CAD build for the part. Positions are in the model's coordinates, mm. A direction names the side the tool comes from. Coordinates: 2 decimals unless noted, no trailing zeros. Loops run counter-clockwise (first coordinate to the right, second up) from the corner with the lowest first, then second, coordinate; pieces in that order, holes last. Notation, with made-up numbers: (-16, 35.5) - (20, 35.5) arc R27 ccw to (20, 73.5) - close; hole circle Ø9 at (-13.5, -34.5). An arc over 180 degrees is marked (long way). Put each result on its own line as item: value.
Autodesk Inventor part; units mm, degrees
ref_plane "YZ Plane" through (0, 0, 0) normal (1, 0, 0) x (0, 1, 0)
ref_plane "XZ Plane" through (0, 0, 0) normal (0, 1, 0) x (-1, 0, 0)
ref_plane "XY Plane" through (0, 0, 0) normal (0, 0, 1) x (1, 0, 0)
sketch "スケッチ1" plane through (0, 0, 0) normal (0, 0, 1) x (1, 0, 0)
  line L0 (29.75, 17.5) -> (29.75, -17.5)
  line L1 (29.75, -17.5) -> (-29.75, -17.5)
  line L2 (-29.75, -17.5) -> (-29.75, 17.5)
  line L3 (-29.75, 17.5) -> (29.75, -17.5) construction
  line L4 (29.75, 17.5) -> (-29.75, -17.5) construction
  line L5 (-3.4667, -15.05) -> (-1.3667, -15.05) construction
  line L6 (15.4667, -15.05) -> (15.4667, -12.45)
  line L7 (15.4667, -12.45) -> (13.3667, -12.45) construction
  line L8 (-3.4667, -12.45) -> (-3.4667, -15.05)
  line L9 (-3.4667, -15.05) -> (15.4667, -12.45) construction
  line L10 (15.4667, -15.05) -> (-3.4667, -12.45) construction
  line L11 (-3.4167, -12.5) -> (15.4167, -12.5) construction
  line L12 (15.4167, -12.5) -> (15.4167, -15) construction
  line L13 (15.4167, -15) -> (-3.4167, -15) construction
  line L14 (-3.4167, -15) -> (-3.4167, -12.5) construction
  line L15 (-3.4167, -12.5) -> (15.4167, -15) construction
  line L16 (15.4167, -12.5) -> (-3.4167, -15) construction
  arc A0 (-1.3667, -12.45) -> (-3.4667, -12.45) centre (-2.4167, -12.45) ccw
  line L17 (-3.4667, -13.75) -> (15.4667, -13.75) construction
  arc A1 (-3.4667, -15.05) -> (-1.3667, -15.05) centre (-2.4167, -15.05) ccw
  line L18 (-1.3667, -12.45) -> (-3.4667, -12.45) construction
  line L19 (-1.3667, -15.05) -> (13.3667, -15.05)
  line L20 (13.3667, -12.45) -> (-1.3667, -12.45)
  line L21 (13.3667, -15.05) -> (15.4667, -15.05) construction
  line L22 (-29.75, 17.5) -> (29.75, 17.5)
  line L23 (6, 17.5) -> (6, -17.5) construction
  line L24 (-29.75, 0) -> (29.75, 0) construction
  arc A2 (15.4667, -12.45) -> (13.3667, -12.45) centre (14.4167, -12.45) ccw
  arc A3 (13.3667, -15.05) -> (15.4667, -15.05) centre (14.4167, -15.05) ccw
  line L25 (-3.4667, 15.05) -> (-1.3667, 15.05) construction
  line L26 (15.4667, 15.05) -> (15.4667, 12.45)
  line L27 (15.4667, 12.45) -> (13.3667, 12.45) construction
  line L28 (-3.4667, 12.45) -> (-3.4667, 15.05)
  line L29 (-3.4667, 15.05) -> (15.4667, 12.45) construction
  line L30 (15.4667, 15.05) -> (-3.4667, 12.45) construction
  line L31 (-3.4167, 12.5) -> (15.4167, 12.5) construction
  line L32 (15.4167, 12.5) -> (15.4167, 15) construction
  line L33 (15.4167, 15) -> (-3.4167, 15) construction
  line L34 (-3.4167, 15) -> (-3.4167, 12.5) construction
  line L35 (-3.4167, 12.5) -> (15.4167, 15) construction
  line L36 (15.4167, 12.5) -> (-3.4167, 15) construction
  arc A4 (-3.4667, 12.45) -> (-1.3667, 12.45) centre (-2.4167, 12.45) ccw
  line L37 (-3.4667, 13.75) -> (15.4667, 13.75) construction
  arc A5 (-1.3667, 15.05) -> (-3.4667, 15.05) centre (-2.4167, 15.05) ccw
  line L38 (-1.3667, 12.45) -> (-3.4667, 12.45) construction
  line L39 (-1.3667, 15.05) -> (13.3667, 15.05)
  line L40 (13.3667, 12.45) -> (-1.3667, 12.45)
  line L41 (13.3667, 15.05) -> (15.4667, 15.05) construction
  arc A6 (15.4667, 15.05) -> (13.3667, 15.05) centre (14.4167, 15.05) ccw
  arc A7 (13.3667, 12.45) -> (15.4667, 12.45) centre (14.4167, 12.45) ccw
  circle A8 centre (25.4167, -12.5) radius 1.6
  circle A9 centre (25.4167, -12.5) radius 3
  circle A10 centre (25.4167, 12.5) radius 1.6
  circle A11 centre (25.4167, 12.5) radius 3
  circle A12 centre (-24.75, 12.5) radius 1.6
  circle A13 centre (-24.75, 12.5) radius 3
  line L42 (-5.9667, -15) -> (-5.9667, -8.9)
  line L43 (-5.9667, -8.9) -> (21.2585, -8.9)
  line L44 (27.25, -7.3146) -> (27.25, 7.3146)
  line L45 (-19.851, 15) -> (-5.9167, 15)
  arc A14 (-21.15, 8.3419) -> (-19.851, 15) centre (-24.75, 12.5) ccw
  line L46 (-27.25, 2.5) -> (-24.75, 2.5) construction
  line L47 (-24.75, 2.5) -> (-24.75, -7.5) construction
  line L48 (-24.75, -7.5) -> (-27.25, -7.5) construction
  line L49 (-27.25, -7.5) -> (-27.25, 2.5) construction
  line L50 (-27.25, 2.5) -> (-24.75, -7.5) construction
  line L51 (-24.75, 2.5) -> (-27.25, -7.5) construction
  line L52 (-27.3, 2.55) -> (-24.7, 2.55)
  line L53 (-24.7, 2.55) -> (-24.7, -7.55)
  line L54 (-24.7, -7.55) -> (-27.3, -7.55)
  line L55 (-27.3, -7.55) -> (-27.3, 2.55)
  line L56 (-27.3, 2.55) -> (-24.7, -7.55) construction
  line L57 (-24.7, 2.55) -> (-27.3, -7.55) construction
  arc A15 (-27.3, 2.55) -> (-27.3, 0.45) centre (-27.3, 1.5) ccw
  line L58 (-26, 2.55) -> (-26, -7.55) construction
  line L59 (-27.3, -2.5) -> (-24.7, -2.5) construction
  arc A16 (-24.7, 0.45) -> (-24.7, 2.55) centre (-24.7, 1.5) ccw
  arc A17 (-27.3, -5.45) -> (-27.3, -7.55) centre (-27.3, -6.5) ccw
  arc A18 (-24.7, -7.55) -> (-24.7, -5.45) centre (-24.7, -6.5) ccw
  line L60 (-21.15, 8.3419) -> (-21.15, -15)
  line L61 (-5.9667, 15) -> (-5.9667, 8.9)
  line L62 (-21.15, -15) -> (-5.9667, -15)
  arc A19 (27.25, -7.3146) -> (21.2585, -8.9) centre (25.4167, -12.5) ccw
  line L63 (-5.9667, 8.9) -> (21.2585, 8.9)
  arc A20 (21.2585, 8.9) -> (27.25, 7.3146) centre (25.4167, 12.5) ccw
  point P0 (0, 0)
  point P1 (6, -13.75)
  point P2 (6, -13.75)
  point P3 (6, -13.75)
  point P4 (6, 13.75)
  point P5 (6, 13.75)
  point P6 (6, 13.75)
  point P7 (-26, -2.5)
  point P8 (-27.3, -5.45)
  point P9 (-24.7, 0.45)
  point P10 (-24.7, -5.45)
  point P11 (-5.9667, 15)
  point P12 (27.25, 7.3146)
  dimension "d0" = 59.5
  dimension "d1" = 35
  dimension "d6" = 18.8333
  dimension "d7" = 0.05
  dimension "d8" = 0.05
  dimension "d9" = 1.05
  dimension "d26" = 35.75
  dimension "d27" = 5
  dimension "d31" = 3.2
  dimension "d32" = 6
  dimension "d33" = 5
  dimension "d34" = 10
  dimension "d39" = 5
  dimension "d40" = 5
  dimension "d41" = 3.2
  dimension "d42" = 6
  dimension "d43" = 2.5
  dimension "d50" = 2.5
  dimension "d51" = 2.5
  dimension "d54" = 2.5
  dimension "d56" = 2.5
  dimension "d60" = 1.05
  dimension "d61" = 0.05
  dimension "d62" = 0.05
  dimension "d63" = 2.5
  dimension "d64" = 2.5
  dimension "d65" = 10
  dimension "d68" = 2.5
  dimension "d71" = 2.5
  dimension "d75" = 10
  dimension "d76" = 2.5
  dimension "d77" = 2.5
extrude "押し出し1" add sketch "スケッチ1" along normal blind 5 contours L0 L1 L2 L22
extrude "押し出し2" add sketch "スケッチ1" along normal blind 2 contours A9 | A11 | A13
chamfer "面取り1" distance 2.5 angle 45 4 edges at (-29.75, 17.5, 2.5) (-29.75, -17.5, 2.5) (29.75, 17.5, 2.5) (29.75, -17.5, 2.5)
extrude "押し出し3" add sketch "スケッチ1" along normal blind 0.5 contours L62 L60 A14 L45 L61 L63 A20 L44 A19 L43 L42
fillet "フィレット1" radius 1 11 edges at (-19.851, 15, 2.75) (-21.15, 8.3419, 2.75) (-5.9667, -8.9, 2.75) (-5.9667, 15, 2.75) (-5.9667, -15, 2.75) (-21.15, -15, 2.75) (21.2585, 8.9, 2.75) (27.25, 7.3146, 2.75) (27.25, -7.3146, 2.75) (21.2585, -8.9, 2.75) (-5.9667, 8.9, 2.75)
equation "\"d6\" = d4"
equation "\"d8\" = d7"
equation "\"d41\" = d31"
equation "\"d42\" = d32"
equation "\"d50\" = d49"
equation "\"d60\" = d9"
equation "\"d61\" = d7"
equation "\"d62\" = d61"
properties part number "Cockpit_vertical_frame_05" material "アセタール樹脂、黒"
Q1. Tool access for faces 5 (the flat face through (27, 11, 2)), 6 (the flat face through (0, 0, 0)), 7 (the flat face through (-27.3, -3, 2)): list every direction of +Z, -Z, +X, -X, +Y, -Y with a clear straight run to the whole face (end or side of a thin tool).
Determined:
face 5: +Z
face 6: -Z, +X, -X, +Y, -Y
face 7: +Z, -Z
Q2. Slice it at B-B, the plane x = -14.5. Give the cut face in (y, z), then the cut area to 3 significant figures.
Determined:
outline: (-17.5, 0) - (17.5, 0) - (17.5, 5) - (15, 5) - (15, 0.5) - (-15, 0.5) - (-15, 5) - (-17.5, 5) - close
area: 40.0 mm2
Q3. Wall check: L1, parallel to Y at x = 10, z = 1.55; L2, parallel to X at y = -4, z = 1.4; L3, parallel to X at y = 1.5, z = 4.4. Give the ranges that are in metal, low to high. Write a range as from..to.
Determined:
L1: -17.5..-15.05, -12.45..-8.9, 8.9..12.45, 15.05..17.5
L2: -29.75..-27.3, -24.7..-21.15, 27.25..29.75
L3: -29.75..-28.35, -23.65..-21.15, 27.25..29.75
Q4. Mould opens along Y. For faces 1 (the flat face through (-28.52, 16.23, 2.53)), 2 (the cylindrical face through (-23.65, -6.48, 2.46)), 3 (the flat face through (0, -17.5, 2)), 4 (the cylindrical face through (-24.01, 13.92, 0.99)) say: +Y half, -Y half, draft (parallel to the pull), parting line (faces both ways), or undercut.
Determined:
face 1: +Y half
face 2: undercut
face 3: -Y half
face 4: undercut
Q5. Slice it at C-C, the plane z = 3.8. State how many separate pieces and enclosed holes the cut face has, then the cut area to 3 significant figures.
Determined:
separate pieces: 1
enclosed holes: 7
area: 822 mm2
Q6. Pin check, flat tips, straight feed: pin 1 Ø3 at (x, y) = (25.42, -12.5) entering from -Z; pin 2 Ø6.5 at (x, y) = (26, -11) entering from +Z. Stop position of each tip, or through.
Determined:
pin 1: through
pin 2: z = 5
Q7. Slice it at A-A, the plane x = 3. Give the cut face in (y, z).
Determined:
outline: (-17.5, 0) - (-15.05, 0) - (-15.05, 5) - (-17.5, 5) - close; (-12.45, 0) - (12.45, 0) - (12.45, 5) - (8.9, 5) - (8.9, 0.5) - (-8.9, 0.5) - (-8.9, 5) - (-12.45, 5) - close; (15.05, 0) - (17.5, 0) - (17.5, 5) - (15.05, 5) - close
